```python
from build123d import *

# Parameters (mm, degrees)
F0_R      = 12
F1_DEPTH  = 7
F2_R      = 7.5
F3_DEPTH  = 64
F5_D      = 7
F5_DEPTH  = 16
F5_TIP    = 2.1030121666
F6_R      = 12
F6_R_2    = 11
F7_DEPTH  = 0.3
F8_R      = 5.65
F9_DEPTH  = 8
F10_SIZE2 = 1.7320508076
F10_SIZE  = 3
F11_R     = 6.15
F11_R_2   = 5.65
F12_DEPTH = 1
F14_DEPTH = 5
F16_DEPTH = 26


with BuildPart() as f1:
    # F0 (on Front) → F1 (new body)
    with BuildSketch(Plane.XZ):
        Circle(F0_R)
    extrude(amount=F1_DEPTH)

    # F2 (on face) → F3 (join)
    with BuildSketch(Plane(origin=(0, 0, 0), x_dir=(-1, 0, 0), z_dir=(0, 1, 0))):
        Circle(F2_R)
    extrude(amount=F3_DEPTH)

    # F5
    with Locations(Plane(origin=(0, 64, 0), x_dir=(-1, 0, 0), z_dir=(0, 1, 0))):
        with Locations((0, 0)):
            Hole(F5_D / 2, depth=F5_DEPTH)
            with Locations((0, 0, -(F5_DEPTH + F5_TIP / 2))):  # 118° drill point
                Cone(0, F5_D / 2, F5_TIP, mode=Mode.SUBTRACT)

    # F6 (on face) → F7 (cut)
    with BuildSketch(Plane.XZ.offset(7)):
        Circle(F6_R)
        Circle(F6_R_2, mode=Mode.SUBTRACT)
    extrude(amount=-F7_DEPTH, mode=Mode.SUBTRACT)

    # F8 (on face) → F9 (join)
    with BuildSketch(Plane.XZ.offset(7)):
        Circle(F8_R)
    extrude(amount=F9_DEPTH)

    # F10
    f10_edges = [f1.edges().sort_by_distance(p)[0] for p in [
        (-5.65, -15, 0),
    ]]
    f10_side = f1.faces().sort_by_distance((0, -15, 0))[0]
    chamfer(f10_edges, length=F10_SIZE, length2=F10_SIZE2, reference=f10_side)

    # F11 (on face) → F12 (cut)
    with BuildSketch(Plane.XZ.offset(7)):
        Circle(F11_R)
        Circle(F11_R_2, mode=Mode.SUBTRACT)
    extrude(amount=-F12_DEPTH, mode=Mode.SUBTRACT)

    # F13 (on face) → F14 (cut)
    with BuildSketch(Plane.XZ.offset(7)):
        with BuildLine():
            ThreePointArc((-9.375, 7.4906191333), (-12, 0), (-9.375, -7.4906191333))
            ThreePointArc((-9.375, -7.4906191333), (-9.0067811764, -7.148069004), (-8.65625, -6.7874395716))
            ThreePointArc((-8.65625, -6.7874395716), (-11, 0), (-8.65625, 6.7874395716))
            ThreePointArc((-8.65625, 6.7874395716), (-9.0067811764, 7.148069004), (-9.375, 7.4906191333))
        make_face()
        with BuildLine():
            ThreePointArc((-8.65625, 6.7874395716), (-11, 0), (-8.65625, -6.7874395716))
            ThreePointArc((-8.65625, -6.7874395716), (-6.8954530534, -4.1360881152), (-6.056953125, -1.0657480197))
            ThreePointArc((-6.056953125, -1.0657480197), (-6.15, 0), (-6.056953125, 1.0657480197))
            ThreePointArc((-6.056953125, 1.0657480197), (-6.8954530534, 4.1360881152), (-8.65625, 6.7874395716))
        make_face()
        with BuildLine():
            ThreePointArc((-1.0657480197, 6.056953125), (0, 6.15), (1.0657480197, 6.056953125))
            ThreePointArc((1.0657480197, 6.056953125), (4.1360881152, 6.8954530534), (6.7874395716, 8.65625))
            ThreePointArc((6.7874395716, 8.65625), (0, 11), (-6.7874395716, 8.65625))
            ThreePointArc((-6.7874395716, 8.65625), (-4.1360881152, 6.8954530534), (-1.0657480197, 6.056953125))
        make_face()
        with BuildLine():
            ThreePointArc((7.4906191333, 9.375), (0, 12), (-7.4906191333, 9.375))
            ThreePointArc((-7.4906191333, 9.375), (-7.148069004, 9.0067811764), (-6.7874395716, 8.65625))
            ThreePointArc((-6.7874395716, 8.65625), (0, 11), (6.7874395716, 8.65625))
            ThreePointArc((6.7874395716, 8.65625), (7.148069004, 9.0067811764), (7.4906191333, 9.375))
        make_face()
        with BuildLine():
            ThreePointArc((6.056953125, -1.0657480197), (6.8954530534, -4.1360881152), (8.65625, -6.7874395716))
            ThreePointArc((8.65625, -6.7874395716), (10.3975658209, -3.5903516541), (11, 0))
            ThreePointArc((11, 0), (10.3975658209, 3.5903516541), (8.65625, 6.7874395716))
            ThreePointArc((8.65625, 6.7874395716), (6.8954530534, 4.1360881152), (6.056953125, 1.0657480197))
            ThreePointArc((6.056953125, 1.0657480197), (6.1266941216, 0.5349010569), (6.15, 0))
            ThreePointArc((6.15, 0), (6.1266941216, -0.5349010569), (6.056953125, -1.0657480197))
        make_face()
        with BuildLine():
            ThreePointArc((8.65625, -6.7874395716), (9.0067811764, -7.148069004), (9.375, -7.4906191333))
            ThreePointArc((9.375, -7.4906191333), (11.3247516529, -3.9686269666), (12, 0))
            ThreePointArc((12, 0), (11.3247516529, 3.9686269666), (9.375, 7.4906191333))
            ThreePointArc((9.375, 7.4906191333), (9.0067811764, 7.148069004), (8.65625, 6.7874395716))
            ThreePointArc((8.65625, 6.7874395716), (10.3975658209, 3.5903516541), (11, 0))
            ThreePointArc((11, 0), (10.3975658209, -3.5903516541), (8.65625, -6.7874395716))
        make_face()
        with BuildLine():
            ThreePointArc((-6.7874395716, -8.65625), (0, -11), (6.7874395716, -8.65625))
            ThreePointArc((6.7874395716, -8.65625), (4.1360881152, -6.8954530534), (1.0657480197, -6.056953125))
            ThreePointArc((1.0657480197, -6.056953125), (0, -6.15), (-1.0657480197, -6.056953125))
            ThreePointArc((-1.0657480197, -6.056953125), (-4.1360881152, -6.8954530534), (-6.7874395716, -8.65625))
        make_face()
        with BuildLine():
            ThreePointArc((-7.4906191333, -9.375), (0, -12), (7.4906191333, -9.375))
            ThreePointArc((7.4906191333, -9.375), (7.148069004, -9.0067811764), (6.7874395716, -8.65625))
            ThreePointArc((6.7874395716, -8.65625), (0, -11), (-6.7874395716, -8.65625))
            ThreePointArc((-6.7874395716, -8.65625), (-7.148069004, -9.0067811764), (-7.4906191333, -9.375))
        make_face()
    extrude(amount=-F14_DEPTH, mode=Mode.SUBTRACT)

    # F15 (on face) → F16 (cut)
    with BuildSketch(Plane.XZ.offset(15)):
        with BuildLine():
            Line((0, 5.3420297766), (0.3, 5.6420297766))
            ThreePointArc((0.3, 5.6420297766), (0, 5.65), (-0.3, 5.6420297766))
            Line((-0.3, 5.6420297766), (0, 5.3420297766))
        make_face()
        with BuildLine():
            ThreePointArc((-5.6420297766, 0.3), (-5.65, 0), (-5.6420297766, -0.3))
            Line((-5.6420297766, -0.3), (-5.3420297766, 0))
            Line((-5.3420297766, 0), (-5.6420297766, 0.3))
        make_face()
        with BuildLine():
            ThreePointArc((-0.3, -5.6420297766), (0, -5.65), (0.3, -5.6420297766))
            Line((0.3, -5.6420297766), (0, -5.3420297766))
            Line((0, -5.3420297766), (-0.3, -5.6420297766))
        make_face()
        with BuildLine():
            ThreePointArc((5.6420297766, -0.3), (5.65, 0), (5.6420297766, 0.3))
            Line((5.6420297766, 0.3), (5.3420297766, 0))
            Line((5.3420297766, 0), (5.6420297766, -0.3))
        make_face()
    extrude(amount=-F16_DEPTH, mode=Mode.SUBTRACT)


solid = f1.part
```
For this review, take the finished solid that the model builds, in its own axes (mm). A direction names the side the tool comes from. Round coordinates to 2 decimals unless told otherwise and drop trailing zeros. Write each loop counter-clockwise with the first axis right and the second up, starting at its lowest first coordinate (ties: lowest second). Pieces come first, ordered by that corner, then holes. Notation, with made-up numbers: (40.5, 74) - (61.5, 74) arc R18 cw to (61.5, 97) - close; hole circle Ø6 at (13.5, 84.5). An arc over 180 degrees is marked (long way). Answer as a JSON object with one key per item and string values.
1. To check wall thickness, follow line 1 along Z through (x, y) = (0, 52.5); line 2 along Y through (x, z) = (-5, -9.5); line 3 along Y through (x, z) = (-6.25, -2.75). State the ranges of each line that lie inside material, in increasing order.
Response values:
{"line 1": "z = -7.5 to -3.5, 3.5 to 7.5", "line 2": "y = -2 to 0", "line 3": "y = -7 to 64"}
2. For pin 1 Ø2 at (x, z) = (-8.5, -8) entering from -Y; pin 2 Ø6.5 at (x, z) = (-3.5, 8) entering from -Y; pin 3 Ø8 at (x, z) = (8.5, -8.5) entering from +Y; pin 4 Ø1 at (x, y) = (-9.5, 8) entering from +Z, all flat-tipped, find the tip position at first contact; note any pin that passes through.
Response values:
{"pin 1": "stops at y = -7", "pin 2": "stops at y = -13.36", "pin 3": "stops at y = 0", "pin 4": "passes through"}
3. We need section A-A on y = 49.5. Give the boundary of the cut face in (x, z).
Response values:
{"outline": "circle Ø15 at (0, 0); hole circle Ø7 at (0, 0)"}
4. Tool access review of faces 1 (the face through (-6, -7, 5)), 2 (the face through (0, -2, -9)), 3 (the face through (-9, -2, 0)), 4 (the face through (-4.311, -6.507, 4.386)): name each direction out of +Z, -Z, +X, -X, +Y, -Y from which nothing blocks a thin tool from reaching the whole face with its end or side.
Response values:
{"face 1": "+Z, -X, -Y", "face 2": "-Z, -Y", "face 3": "-X, -Y", "face 4": "-Y"}
5. We need section B-B on y = 38. Give the boundary of the cut face in (x, z), then the cut area to 3 significant figures.
Response values:
{"outline": "circle Ø15 at (0, 0)", "area": "177 mm2"}
6. Draft analysis for pull direction Z (two halves, no side actions). For faces 5 (the face through (4.311, -6.507, -4.386)), 6 (the face through (0, -2, 9)), 7 (the face through (4.386, -6.507, 4.311)), 8 (the face through (7.493, 31.552, 0.33)), state which applies: +Z half, -Z half, draft (parallel to the pull), parting line (faces both ways), or undercut.
Response values:
{"face 5": "undercut", "face 6": "draft", "face 7": "undercut", "face 8": "parting line"}
